Source: CAD feature listing. Evaluate the final solid. Frame: model axes, mm. Face numbers are marked on the shaded views. A direction names the side the tool comes from. Round coordinates to 2 decimals unless told otherwise and drop trailing zeros. Order: outer loops, then holes, each group sorted by start corner. A loop starts at its lowest first (then second) coordinate and runs counter-clockwise, first axis right, second up. Notation, with made-up numbers: (2.5, 80.5) - (35.5, 80.5) arc R20 cw to (35.5, 116.5) - close; hole circle Ø11 at (-29, 27). An arc over 180 degrees is marked (long way). Put each result on its own line as item: value. Start each with the question number.
1) Section A-A on x = 7.5. Output: boundary loops of the cut face in (y, z).
2) Section C-C on y = 11.75. Output: boundary loops of the cut face in (x, z).
3) Contact query for a flat-ended pin moving along its axis: P1, Ø1.5, axis at x = 41, y = 4, coming from the +Z side. Output: stop coordinate, or through.
4) Mould query, pull axis X, two halves, no side actions, for the marked faces 3, 4 and 5. Classes: +X half, -X half, draft (parallel to the pull), parting line (faces both ways), or undercut.
5) Section D-D on x = 37. Output: boundary loops of the cut face in (y, z).
6) Access query for the marked faces 1 and 2. Directions: +Z, -Z, +X, -X, +Y, -Y. A direction counts if a zero-diameter tool reaches every point of the face in a straight line with its end or side. Return the directions, or none.
7) Line query: probe 1 along Y at (x, z) = (44, -8.25). Output: solid intervals per line, ascending. Write a range as [from, to].
8) Section B-B on z = -4.5. Output: boundary loops of the cut face in (x, y), then the cut area to 3 significant figures.
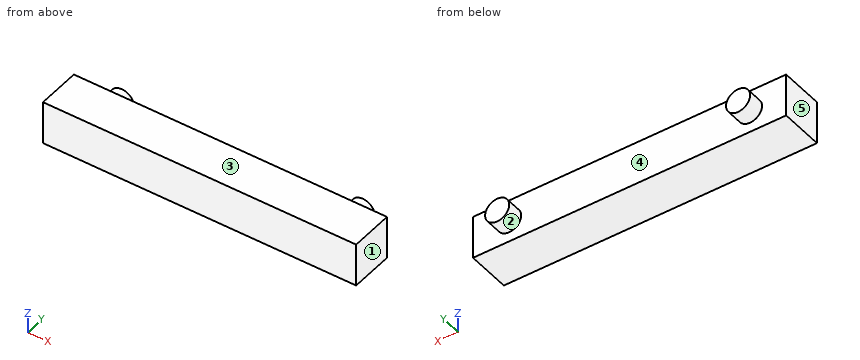
```python
from build123d import *

# Parameters (mm, degrees)
SKETCH1_W           = 65
SKETCH1_H           = 9
BOSS_EXTRUDE1_DEPTH = 9
SKETCH2_R           = 2.5
BOSS_EXTRUDE2_DEPTH = 3.5


with BuildPart() as part:
    # Sketch1 → Boss-Extrude1 (new body)
    with BuildSketch(Plane(origin=(0, 0, 0), x_dir=(1, 0, 0), z_dir=(0, 1, 0))):
        with Locations((32.5, 4.5)):
            Rectangle(SKETCH1_W, SKETCH1_H)
    extrude(amount=BOSS_EXTRUDE1_DEPTH)

    # Sketch2 → Boss-Extrude2 (add)
    with BuildSketch(Plane(origin=(0, 9, 0), x_dir=(1, 0, 0), z_dir=(0, 1, 0))):
        with Locations(Location((7.5, 4.5, 0), (0, 0, 90))):  # turned: the seam where the file's is
            Circle(SKETCH2_R)
        with Locations(Location((57.5, 4.5, 0), (0, 0, 90))):  # turned: the seam where the file's is
            Circle(SKETCH2_R)
    extrude(amount=BOSS_EXTRUDE2_DEPTH)


solid = part.part
```
Answer sheet:
1. outline: (0, -9) - (9, -9) - (9, -7) - (12.5, -7) - (12.5, -2) - (9, -2) - (9, 0) - (0, 0) - close
2. outline: circle Ø5 at (7.5, -4.5); circle Ø5 at (57.5, -4.5)
3. P1: z = 0
4. face 3: draft
4. face 4: undercut
4. face 5: -X half
5. outline: (0, -9) - (9, -9) - (9, 0) - (0, 0) - close
6. face 1: +Z, -Z, +X, +Y, -Y
6. face 2: +Y
7. probe 1: [0, 9]
8. outline: (0, 0) - (65, 0) - (65, 9) - (60, 9) - (60, 12.5) - (55, 12.5) - (55, 9) - (10, 9) - (10, 12.5) - (5, 12.5) - (5, 9) - (0, 9) - close
8. area: 620 mm^2
